Drawing for the job (mm, zero at the part's lowest x, y, z). Coordinates: 2 decimals unless noted, no trailing zeros. Order: outer loops, then holes, each group sorted by start corner. A loop starts at its lowest first (then second) coordinate and runs counter-clockwise, first axis right, second up.
1) Wall check: L1, parallel to Z at x = 12.7, y = 19.75; L2, parallel to Y at x = 22.5, z = 12.7. Give the ranges that are in metal, low to high.
2) Cut at D-D (z = 5.75). List the corners of the cut face in (x, y), and give its area (3 significant figures).
3) Cut at C-C (y = 12.5). List the corners of the cut face in (x, z).
4) Cut at A-A (z = 12.7). List the corners of the cut face in (x, y).
5) Mould opens along X. For the marked faces 1, 2 and 3 say: +X half, -X half, draft (parallel to the pull), parting line (faces both ways), or undercut.
6) Cut at B-B (x = 12.7). List the corners of the cut face in (y, z).
7) Pin check, flat tip, straight feed: pin 1 Ø14 at (x, y) = (12.7, 12.5) entering from -Z. Stop position of the tip, or through.
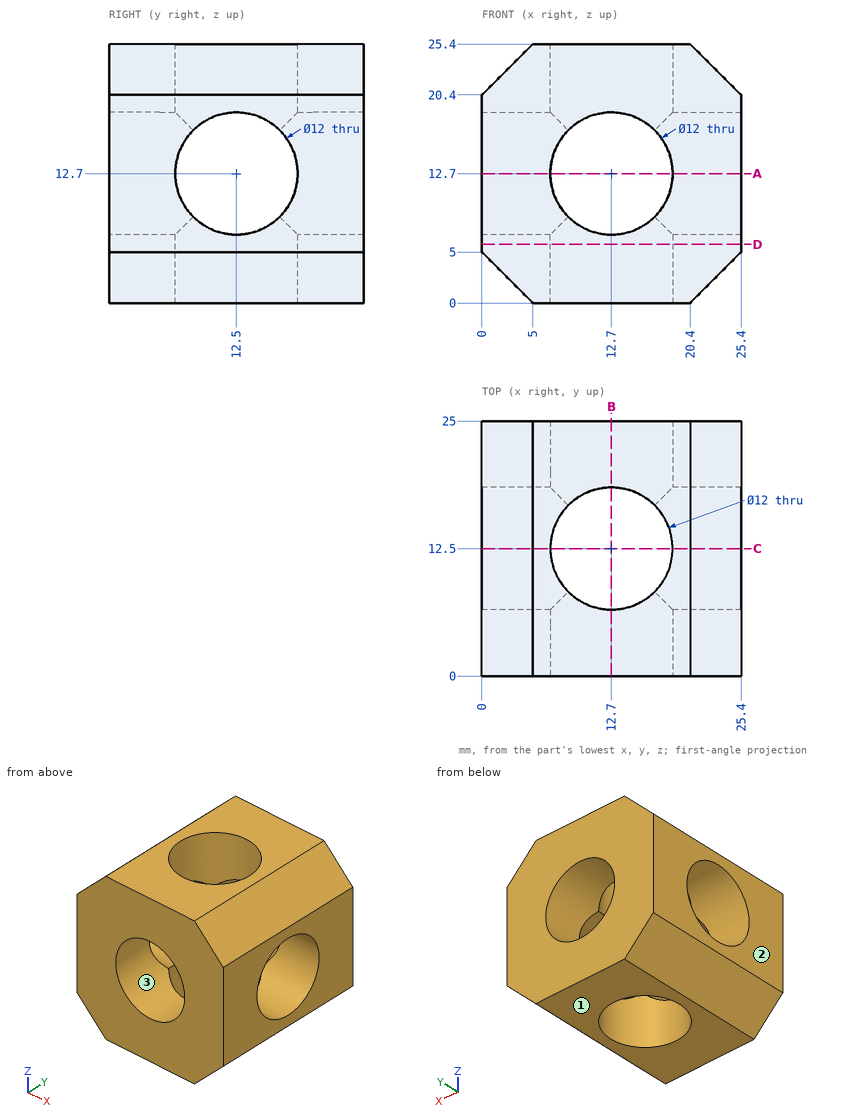
Geometry check:
1. L1: z = 0 to 6.7, 18.7 to 25.4
1. L2: y = 0 to 6.5, 18.5 to 25
2. outline: (0, 0) - (25.4, 0) - (25.4, 25) - (0, 25) - close; hole circle Ø12 at (12.7, 12.5)
2. area: 522 mm2
3. outline: (0, 5) - (5, 0) - (6.7, 0) - (6.7, 6.7) - (0, 6.7) - close; (0, 18.7) - (6.7, 18.7) - (6.7, 25.4) - (5, 25.4) - (0, 20.4) - close; (18.7, 0) - (20.4, 0) - (25.4, 5) - (25.4, 6.7) - (18.7, 6.7) - close; (18.7, 18.7) - (25.4, 18.7) - (25.4, 20.4) - (20.4, 25.4) - (18.7, 25.4) - close
4. outline: (0, 0) - (6.7, 0) - (6.7, 6.5) - (0, 6.5) - close; (0, 18.5) - (6.7, 18.5) - (6.7, 25) - (0, 25) - close; (18.7, 0) - (25.4, 0) - (25.4, 6.5) - (18.7, 6.5) - close; (18.7, 18.5) - (25.4, 18.5) - (25.4, 25) - (18.7, 25) - close
5. face 1: draft
5. face 2: -X half
5. face 3: undercut
6. outline: (0, 0) - (6.5, 0) - (6.5, 6.7) - (0, 6.7) - close; (0, 18.7) - (6.5, 18.7) - (6.5, 25.4) - (0, 25.4) - close; (18.5, 0) - (25, 0) - (25, 6.7) - (18.5, 6.7) - close; (18.5, 18.7) - (25, 18.7) - (25, 25.4) - (18.5, 25.4) - close
7. pin 1: stops at z = 0
